```python
from build123d import *

# Parameters (mm, degrees)
F1_DEPTH = 8
F0_W     = 42
F0_H     = 7
F0_R     = 1.75
F2_DEPTH = 4
F4_R     = 2.5
F5_DEPTH = 20.001


# Not quite as in the source:
# - a fillet or chamfer that OpenCascade refuses, or shapes differently, is made with other operations: its cross-section is extruded or revolved along the edge and cut away or added


with BuildPart() as f1:
    # F0 (on Top) → F1 (new body)
    with BuildSketch(Plane.XY):
        Polygon((0, -6.5), (0, 0), (0, 7), (0, 13.5), (-8, 13.5), (-8, -6.5), align=None)
    extrude(amount=F1_DEPTH)

    # F0 (on Top) → F2 (join)
    with BuildSketch(Plane.XY):
        with Locations((21, 3.5)):
            Rectangle(F0_W, F0_H)
        with Locations((38.5, 3.5)):
            Circle(F0_R, mode=Mode.SUBTRACT)
    extrude(amount=F2_DEPTH)

    # F3: fillet of radius 2 on 2 edges, made by hand

    # F3_s1 → F3_t2 (revolve, cut)
    with BuildSketch(Plane.XZ.offset(-3.5)):
        with BuildLine():
            ThreePointArc((42.25, 4), (40.8357864376, 3.4142135624), (40.25, 2))
            Line((40.25, 2), (40.25, 4))
            Line((40.25, 4), (42.25, 4))
        make_face()
    revolve(axis=Axis((38.5, 3.5, 4), (0, 0, 1)), mode=Mode.SUBTRACT)

    # F3_s3 → F3_t4 (revolve, cut)
    with BuildSketch(Plane.XZ.offset(-3.5)):
        with BuildLine():
            ThreePointArc((42.25, 0), (40.8357864376, 0.5857864376), (40.25, 2))
            Line((40.25, 2), (40.25, 0))
            Line((40.25, 0), (42.25, 0))
        make_face()
    revolve(axis=Axis((38.5, 3.5, 0), (0, 0, 1)), mode=Mode.SUBTRACT)

    # F4 (on face) → F5 (cut, through all)
    with BuildSketch(Plane.XZ.offset(6.5)):
        with Locations((-4, 4)):
            Circle(F4_R)
    extrude(amount=-F5_DEPTH, mode=Mode.SUBTRACT)


solid = f1.part
```
Geometry: final body of the model. Coordinates: model frame, mm. A direction names the side the tool comes from. Coordinates: 2 decimals unless noted, no trailing zeros. Order: outer loops, then holes, each group sorted by start corner. A loop starts at its lowest first (then second) coordinate and runs counter-clockwise, first axis right, second up. Notation, with made-up numbers: (22.5, 78) - (67.5, 78) arc R24 ccw to (67.5, 110) - close; hole circle Ø11 at (80.25, 23.5). An arc over 180 degrees is marked (long way). Write each question's results on one line, items separated by ' | '.
1) Pull-direction query (X, two-part tool) for faces 1 (the cylindrical face through (-1.615, 3.36, 4.751)), 2 (the flat face through (0, 3, 5)), 3 (the flat face through (41.4, 6.4, 4)); classes: pulls with the +X half, pulls with the -X half, needs draft (parallel to the pull), parting line crosses it, or undercut.
Results list:
face 1: undercut | face 2: pulls with the +X half | face 3: needs draft
2) Pin query (flat end, axial travel): pin 1 (4.5 mm diameter, centred on x = 16, z = 3, fed in from +Y); pin 2 (7.5 mm diameter, centred on x = 16.5, y = 3.5, fed in from +Z); pin 3 (4.5 mm diameter, centred on x = 14.5, z = 2, fed in from -Y). Return the tip coordinate at first contact, or that it passes through.
Results list:
pin 1: y = 7 | pin 2: z = 4 | pin 3: y = 0
3) Set-up query: faces 4 (the flat face through (21, 0, 2)), 5 (the flat face through (41.4, 0.7, 4)), 6 (the flat face through (21, 7, 2)). Return all of +Z, -Z, +X, -X, +Y, -Y with unobstructed straight access to the full face (end or side cutting, diameter ignored); none if empty.
Results list:
face 4: +Z, -Z, +X, -Y | face 5: +Z, +X, +Y, -Y | face 6: +Z, -Z, +X, +Y
4) Section A-A, the plane x = -4. Return loops of the section in (y, z).
Results list:
outline: (-6.5, 0) - (13.5, 0) - (13.5, 1.5) - (-6.5, 1.5) - close; (-6.5, 6.5) - (13.5, 6.5) - (13.5, 8) - (-6.5, 8) - close
5) Section B-B, the plane y = -2.5. Return loops of the section in (x, z).
Results list:
outline: (-8, 0) - (0, 0) - (0, 8) - (-8, 8) - close; hole circle Ø5 at (-4, 4)
6) Line query: line 1 (Z direction, x = -4, y = 7.5); line 2 (Y direction, x = 24.5, z = 1.75); line 3 (X direction, y = 1.5, z = 6). Output: solid intervals per line, ascending. Write a range as from..to.
Results list:
line 1: 0..1.5, 6.5..8 | line 2: 0..7 | line 3: -8..-5.5, -2.5..0
7) Section C-C, the plane x = 29. Return loops of the section in (y, z).
Results list:
outline: (0, 0) - (7, 0) - (7, 4) - (0, 4) - close
